Part model, mm, in its own coordinate system. Face numbers are marked on the shaded views. A direction names the side the tool comes from. Round coordinates to 2 decimals unless told otherwise and drop trailing zeros. Write each loop counter-clockwise with the first axis right and the second up, starting at its lowest first coordinate (ties: lowest second). Pieces come first, ordered by that corner, then holes. Notation, with made-up numbers: M 20,69.25 L 38,69.25 A9 ccw 38,80.25 Z; hole C 63,4.5 d5. An arc over 180 degrees is marked long. Use a Markdown table: item, result. Add a question column.
1) Drop flat-ended pins along their axis: P1, Ø2, axis at y = -2.5, z = 35, coming from the +X side; P2, Ø3, axis at y = 7, z = 15, coming from the -X side; P3, Ø8, axis at x = -7, z = 66, coming from the +Y side. Give the stop position or say it passes through.
2) Wall check: probe 1 along Y at (x, z) = (0, 28); probe 2 along Z at (x, y) = (-4.25, -8); probe 3 along Z at (x, y) = (8, -2.5). Give the ranges that are in metal, low to high.
3) Which spindle directions (+Z, -Z, +X, -X, +Y, -Y) get a long thin tool onto all of the face, cutting with end or side? Do the marked faces 1 and 2. Say none if no direction does.
4) Slice it at D-D on y = 7. Write the cut outline in (x, z), plus the area to 3 significant figures.
5) Slice it at C-C on z = 24.5. Write the cut outline in (x, y), plus the area to 3 significant figures.
6) Slice it at A-A on x = 0. Write the cut outline in (y, z), plus the area to 3 significant figures.
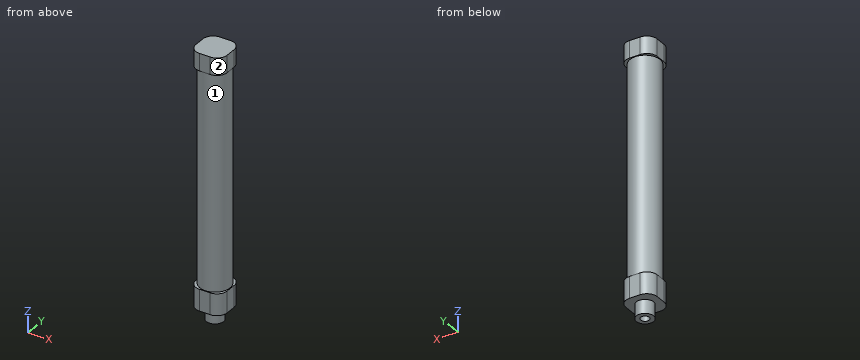
Autodesk Inventor part; units mm, degrees
ref_plane "YZ Plane" through (0, 0, 0) normal (1, 0, 0) x (0, 1, 0)
ref_plane "XZ Plane" through (0, 0, 0) normal (0, 1, 0) x (-1, 0, 0)
ref_plane "XY Plane" through (0, 0, 0) normal (0, 0, 1) x (1, 0, 0)
sketch "スケッチ1" plane through (0, 0, 0) normal (0, 0, 1) x (1, 0, 0)
  line L0 (9.15, -9.15) -> (-9.15, -9.15)
  line L1 (-9.15, -9.15) -> (-9.15, 9.15)
  line L2 (-9.15, 9.15) -> (9.15, 9.15)
  line L3 (9.15, 9.15) -> (9.15, -9.15)
  line L4 (9.15, -9.15) -> (-9.15, 9.15) construction
  line L5 (-9.15, -9.15) -> (9.15, 9.15) construction
  point P0 (0, 0)
  dimension "d0" = 18.3
  dimension "d1" = 18.3
extrude "押し出し1" add sketch "スケッチ1" along normal blind 12.5
sketch "スケッチ2" plane through (0, 0, 12.5) normal (0, 0, 1) x (1, 0, 0)
  circle A0 centre (0, 0) radius 8.75
  dimension "d4" = 17.5
extrude "押し出し2" add sketch "スケッチ2" along normal blind 125
sketch "スケッチ3" plane through (0, 0, 137.5) normal (0, 0, 1) x (1, 0, 0)
  line L0 (-9.15, -9.15) -> (9.15, -9.15)
  line L1 (9.15, -9.15) -> (9.15, 9.15)
  line L2 (9.15, 9.15) -> (-9.15, 9.15)
  line L3 (-9.15, 9.15) -> (-9.15, -9.15)
  line L4 (-9.15, -9.15) -> (9.15, 9.15) construction
  line L5 (9.15, -9.15) -> (-9.15, 9.15) construction
  point P0 (0, 0)
  dimension "d7" = 18.3
  dimension "d8" = 18.3
extrude "押し出し3" add sketch "スケッチ3" along normal blind 10
fillet "フィレット1" radius 6 4 edges at (9.15, 9.15, 142.5) (9.15, -9.15, 142.5) (-9.15, 9.15, 142.5) (-9.15, -9.15, 142.5)
fillet "フィレット2" radius 6 4 edges at (9.15, 9.15, 6.25) (9.15, -9.15, 6.25) (-9.15, 9.15, 6.25) (-9.15, -9.15, 6.25)
sketch "スケッチ4" plane through (0, 0, 0) normal (0, 0, -1) x (-1, 0, 0)
  circle A0 centre (0, 0) radius 5
  dimension "d13" = 10
extrude "押し出し4" add sketch "スケッチ4" along normal blind 8
sketch "スケッチ5" plane through (0, 0, -8) normal (0, 0, -1) x (-1, 0, 0)
  circle A0 centre (0, 0) radius 2.5
  dimension "d16" = 5
extrude "押し出し5" cut sketch "スケッチ5" against normal blind 100
properties part number "aircylinder16_100_part1_sa" material "アルミニウム 6061-AHC"
Entries:
| question | item | result |
|---|---|---|
| 1 | P1 | stops at x = 8.62 |
| 1 | P2 | stops at x = -6.81 |
| 1 | P3 | stops at y = 8.22 |
| 2 | probe 1 | y = -8.75 to -2.5, 2.5 to 8.75 |
| 2 | probe 2 | z = 0 to 12.5, 137.5 to 147.5 |
| 2 | probe 3 | z = 0 to 147.5 |
| 3 | face 1 | none |
| 3 | face 2 | +Z, -Z, +X, -Y |
| 4 | outline | M -7.75,0 L 7.75,0 L 7.75,12.5 L 5.25,12.5 L 5.25,137.5 L 7.75,137.5 L 7.75,147.5 L -7.75,147.5 L -7.75,137.5 L -5.25,137.5 L -5.25,12.5 L -7.75,12.5 Z |
| 4 | area | 1,660 mm^2 |
| 5 | outline | C 0,0 d17.5; hole C 0,0 d5 |
| 5 | area | 221 mm^2 |
| 6 | outline | M -9.15,0 L -5,0 L -5,-8 L -2.5,-8 L -2.5,92 L 2.5,92 L 2.5,-8 L 5,-8 L 5,0 L 9.15,0 L 9.15,12.5 L 8.75,12.5 L 8.75,137.5 L 9.15,137.5 L 9.15,147.5 L -9.15,147.5 L -9.15,137.5 L -8.75,137.5 L -8.75,12.5 L -9.15,12.5 Z |
| 6 | area | 2,180 mm^2 |
